Autodesk Inventor part; units mm, degrees
ref_plane "YZ Plane" through (0, 0, 0) normal (1, 0, 0) x (0, 1, 0)
ref_plane "XZ Plane" through (0, 0, 0) normal (0, 1, 0) x (-1, 0, 0)
ref_plane "XY Plane" through (0, 0, 0) normal (0, 0, 1) x (1, 0, 0)
sketch "Sketch1" plane through (0, 0, 0) normal (0, 0, 1) x (1, 0, 0)
  line L0 (50, 188.2731) -> (-50, 188.2731)
  line L1 (-50, 188.2731) -> (-50, 158.2731)
  line L2 (50, 158.2731) -> (50, 188.2731)
  line L3 (11, 158.2731) -> (11, 174.2731)
  line L4 (11, 174.2731) -> (-11, 174.2731)
  line L5 (-11, 174.2731) -> (-11, 158.2731)
  line L6 (17, 158.2731) -> (17, 180.2731)
  line L7 (17, 180.2731) -> (-17, 180.2731)
  line L8 (-17, 180.2731) -> (-17, 158.2731)
  line L9 (17, 158.2731) -> (50, 158.2731)
  line L10 (11, 158.2731) -> (17, 158.2731)
  line L11 (-11, 158.2731) -> (-17, 158.2731)
  line L12 (-17, 158.2731) -> (-50, 158.2731)
  circle A0 centre (23.5, 173.2731) radius 2.125
  circle A1 centre (-23.5, 173.2731) radius 2.125
  line L13 (0, 0) -> (0, 215.8038) construction
  line L14 (0, 158.2731) -> (11, 158.2731) construction
  line L15 (0, 158.2731) -> (-11, 158.2731) construction
  line L16 (-23.5, 173.2731) -> (23.5, 173.2731) construction
  line L17 (-23.5, 173.2731) -> (-23.5, 188.2731) construction
  line L18 (-23.5, 173.2731) -> (-23.5, 158.2731) construction
  dimension "d1" = 30
  dimension "d2" = 100
  dimension "d3" = 22
  dimension "d4" = 6
  dimension "d5" = 16
  dimension "d6" = 6
  dimension "d11" = 4.25
  dimension "d13" = 4.25
  dimension "d18" = 47
extrude "Extrusion1" add sketch "Sketch1" along normal blind 6 contours L2 L9 L6 L7 L8 L12 L1 L0
extrude "Extrusion2" add sketch "Sketch1" along normal blind 30 contours L10 L3 L4 L5 L11 L8 L7 L6
sketch "Sketch2" plane through (-17, 180.2731, 6) normal (0, 1, 0) x (1, 0, 0)
  circle A0 centre (16.8713, -6) radius 2.125
  line L0 (16.8713, -6) -> (33.9314, -6) construction
  line L1 (16.8713, -6) -> (-0.1889, -6) construction
  line L2 (67, 6) -> (-33, 6)
  point P0 (17, 6)
  dimension "d14" = 4.25
  dimension "d15" = 12
extrude "Extrusion3" cut sketch "Sketch2" against normal up to next
sketch "Sketch3" plane through (0, 0, 6) normal (0, 0, 1) x (1, 0, 0)
  line L0 (50, 158.2731) -> (50, 188.2731)
  line L1 (50, 180.2731) -> (35, 180.2731)
  line L2 (35, 180.2731) -> (35, 166.2731)
  line L3 (35, 166.2731) -> (50, 166.2731)
  line L4 (43.2299, 188.2731) -> (43.2299, 180.2731) construction
  line L5 (43.4666, 166.2731) -> (43.4666, 158.2731) construction
  line L6 (50, 188.2731) -> (-50, 188.2731)
  line L7 (17, 158.2731) -> (50, 158.2731)
  line L8 (-50, 188.2731) -> (-50, 158.2731)
  line L9 (-50, 180.2731) -> (-35, 180.2731)
  line L10 (-35, 180.2731) -> (-35, 166.2731)
  line L11 (-35, 166.2731) -> (-50, 166.2731)
  line L12 (-50, 166.2731) -> (-50, 180.2731)
  point P0 (0, 0)
  dimension "d19" = 15
  dimension "d20" = 14
extrude "Extrusion4" add sketch "Sketch3" along normal blind 25
sketch "Sketch4" plane through (35, 180.2731, 6) normal (0, 1, 0) x (1, 0, 0)
  circle A0 centre (7.5, -10) radius 4
  line L0 (7.5, -10) -> (15, -10) construction
  line L1 (15, 0) -> (15, -25)
  line L2 (7.5, -10) -> (0, -10) construction
  line L3 (0, 0) -> (0, -25)
  line L4 (15, 6) -> (-85, 6)
  line L5 (8, -13.9686) -> (8, -25)
  line L6 (7, -13.9686) -> (7, -25)
  line L7 (8, -37.8452) -> (15, -37.8452) construction
  line L8 (7, -37.8452) -> (0, -37.8452) construction
  circle A1 centre (-77.5, -10) radius 4
  line L9 (-85, -25) -> (-70, -25)
  line L10 (-78, -13.9686) -> (-78, -25)
  line L11 (-77, -37.6694) -> (-70, -37.6694) construction
  line L12 (-78, -37.628) -> (-85, -37.628) construction
  line L13 (-85, 0) -> (-85, -25)
  line L14 (-70, 0) -> (-70, -25)
  line L15 (-77, -13.9686) -> (-77, -25)
  line L16 (-77.5, -10) -> (-70, -10) construction
  line L17 (-77.5, -10) -> (-85, -10) construction
  line L18 (-77, -25) -> (-78, -25)
  line L19 (8, -25) -> (7, -25)
  line L20 (0, -25) -> (15, -25)
  point P0 (-35, 6)
  dimension "d23" = 8
  dimension "d24" = 16
  dimension "d25" = 1
  dimension "d26" = 8
  dimension "d27" = 1
extrude "Extrusion5" cut sketch "Sketch4" against normal up to next
sketch "Sketch5" plane through (-50, 158.2731, 0) normal (-1, 0, 0) x (0, 0, 1)
  circle A0 centre (25.4843, 15) radius 2.125
  line L0 (0, 30) -> (0, 0)
  line L1 (25.4843, 15) -> (25.4843, 22)
  line L2 (6, 22) -> (31, 22)
  line L3 (25.4843, 15) -> (25.4843, 8)
  line L4 (6, 8) -> (31, 8)
  line L5 (25.4843, 15) -> (19.9686, 15)
  line L6 (25.4843, 15) -> (31, 15)
  line L7 (31, 22) -> (31, 8)
  line L8 (19.9686, 22) -> (19.9686, 8)
  point P0 (0, -158.2731)
  dimension "d30" = 4.25
extrude "Extrusion6" cut sketch "Sketch5" against normal up to surface (15 mm away) contours L6 L1 A0 | A0 L3 L6 | L1 L5 A0 | A0 L5 L3
sketch "Sketch6" plane through (50, 158.2731, 0) normal (1, 0, 0) x (0, 0, -1)
  circle A0 centre (-25.4843, 15) radius 2.125
  point P0 (0, -158.2731)
extrude "Extrusion7" cut sketch "Sketch6" against normal up to surface (15 mm away)
properties part number "YPulleySupportBase"
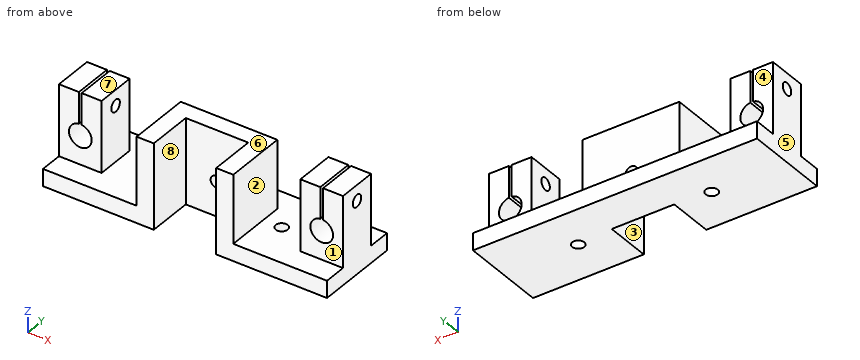
Geometry check sheet. Reference: the model listing, model coordinates, mm. Face numbers are marked on the shaded views. A direction names the side the tool comes from. Round coordinates to 2 decimals unless told otherwise and drop trailing zeros. Loops run counter-clockwise (first coordinate to the right, second up) from the corner with the lowest first, then second, coordinate; pieces in that order, holes last. Notation, with made-up numbers: (88, 45.5) - (112, 45.5) arc R19 cw to (112, 67.5) - close; hole circle Ø5 at (-24.75, 22.25). An arc over 180 degrees is marked (long way). Use a Markdown table: item, result.
Q1. Access from +Z, -Z, +X, -X, +Y, -Y to the whole of each face (thin tool, end or side, straight path). Record for the marked faces 1, 2, 3 and 4.
Solutions:
| item | result |
|---|---|
| face 1 | +Z, +X, -Y |
| face 2 | +Z, +Y, -Y |
| face 3 | +Z, -Z, -Y |
| face 4 | +Z, +X, -X, +Y |
Q2. Material ranges on line 1 (X direction, y = 168.25, z = 11); line 2 (Y direction, x = 23.5, z = 1.55); line 3 (X direction, y = 171, z = 19.5), recorded low to high.
Solutions:
| item | result |
|---|---|
| line 1 | x = -50 to -35, -17 to -11, 11 to 17, 35 to 50 |
| line 2 | y = 158.27 to 171.15, 175.4 to 188.27 |
| line 3 | x = -50 to -44.44, -40.56 to -35, -17 to -11, 11 to 17, 35 to 40.56, 44.44 to 50 |
Q3. Draft check along X on the marked faces 5, 6, 7 and 8. Enter one of: released by +X, released by -X, zero draft, split by the parting line, or undercut.
Solutions:
| item | result |
|---|---|
| face 5 | released by -X |
| face 6 | undercut |
| face 7 | zero draft |
| face 8 | undercut |
Q4. Go/stop test with flat-tipped pins: P1, Ø5.5, axis at x = -23.5, y = 173.27, coming from the +Z side; P2, Ø12, axis at x = 45, z = 14.5, coming from the +Y side. Record where each tip stops, or that it passes through.
Solutions:
| item | result |
|---|---|
| P1 | stops at z = 6 |
| P2 | stops at y = 180.27 |
Q5. Cross-section at B-B on z = 16. Record the cut outline in (x, y).
Solutions:
| item | result |
|---|---|
| outline | (-50, 166.27) - (-46.5, 166.27) - (-46.5, 180.27) - (-50, 180.27) - close; (-38.5, 166.27) - (-35, 166.27) - (-35, 180.27) - (-38.5, 180.27) - close; (-17, 158.27) - (-11, 158.27) - (-11, 174.27) - (11, 174.27) - (11, 158.27) - (17, 158.27) - (17, 180.27) - (-17, 180.27) - close; (35, 166.27) - (38.5, 166.27) - (38.5, 180.27) - (35, 180.27) - close; (46.5, 166.27) - (50, 166.27) - (50, 180.27) - (46.5, 180.27) - close |
Q6. Cross-section at A-A on y = 170.25. Record the cut outline in (x, z).
Solutions:
| item | result |
|---|---|
| outline | (-50, 0) - (-11, 0) - (-11, 30) - (-17, 30) - (-17, 6) - (-35, 6) - (-35, 31) - (-42, 31) - (-42, 19.97) arc R4 cw (long way) to (-43, 19.97) - (-43, 31) - (-50, 31) - close; (11, 0) - (50, 0) - (50, 31) - (43, 31) - (43, 19.97) arc R4 cw (long way) to (42, 19.97) - (42, 31) - (35, 31) - (35, 6) - (17, 6) - (17, 30) - (11, 30) - close |
Q7. Cross-section at D-D on x = 3.5. Record the cut outline in (y, z), plus the area to 3 significant figures.
Solutions:
| item | result |
|---|---|
| outline | (174.27, 0) - (188.27, 0) - (188.27, 6) - (180.27, 6) - (180.27, 30) - (174.27, 30) - close |
| area | 228 mm2 |
Q8. Cross-section at C-C on x = 23.5. Record the cut outline in (y, z).
Solutions:
| item | result |
|---|---|
| outline | (158.27, 0) - (171.15, 0) - (171.15, 6) - (158.27, 6) - close; (175.4, 0) - (188.27, 0) - (188.27, 6) - (175.4, 6) - close |
